Can you work these out from the model? Positions are in its coordinate system, mm. A direction names the side the tool comes from. Coordinates: 2 decimals unless noted, no trailing zeros. Order: outer loops, then holes, each group sorted by start corner. A loop starts at its lowest first (then second) coordinate and runs counter-clockwise, first axis right, second up. Notation, with made-up numbers: (5.25, -30.5) -> (19.25, -30.5) arc R27 cw to (19.25, -1.5) -> close; hole circle Ø3 at (36.25, 83). An arc over 180 degrees is marked (long way). Answer as a JSON object with one key per item and string values. Group by question number.
(1) I want a section at B-B, the plane x = -106. List the corners of the cut face in (y, z) for me, plus the area to 3 significant figures.
(2) If we mould it in two halves opening along X, with no side actions, what happens to faces 4 (the cylindrical face through (-622.038, 0.279, 0.178)), 5 (the flat face through (0, -5.4, 3.64)), 6 (the flat face through (-640, 17, 12.7))? For each: pulls with the +X half, pulls with the -X half, needs draft (parallel to the pull), parting line crosses it, or undercut.
(3) I need wall thicknesses on line 1 (X direction, y = -15, z = 7); line 2 (X direction, y = 7, z = -3.5); line 3 (X direction, y = 7, z = -1.5) (3 decimals). Which ranges of each line are inside material? Lowest first, please.
(4) For pin 1 (4 mm diameter, centred on x = 5, z = -3.5, fed in from -Y); pin 2 (4 mm diameter, centred on y = -14.5, z = -9, fed in from +X); pin 3 (2 mm diameter, centred on x = -356, z = 4, fed in from -Y), each with a flat end and sliding along its axis, tell me the tip position at first contact or that it passes through.
(5) Which directions (+Z, -Z, +X, -X, +Y, -Y) give clear straight access to the entire face, cutting with the end or side of a thin tool? Please do faces 1 (the cylindrical face through (15.51, -11.07, 2.38)), 2 (the cylindrical face through (-300.53, -1.38, -6.2)), 3 (the flat face through (-658, -12.7, 0)).
from build123d import *

# Parameters (mm, degrees)
F0_R     = 6.35
F1_DEPTH = 609.6
F2_W     = 15.875
F2_H     = 15.875
F3_DEPTH = 15.875
F4_R     = 7.9375
F5_DEPTH = 6.35
F6_R     = 6.35
F8_DEPTH = 12.7
F9_R     = 9.525
F10_R    = 3.175


with BuildPart() as f1:
    # F0 (on Right) → F1 (new body)
    with BuildSketch(Plane.YZ):
        Circle(F0_R)
    extrude(amount=-F1_DEPTH)

    # F2 (on Right) → F3 (join)
    with BuildSketch(Plane.YZ):
        Rectangle(F2_W, F2_H)
    extrude(amount=F3_DEPTH)

    # F4 (on face) → F5 (join)
    with BuildSketch(Plane.XZ.offset(7.9375)):
        with Locations((7.9375, 0)):
            Circle(F4_R)
    extrude(amount=F5_DEPTH)

    # F6
    f6_edges = [f1.edges().sort_by_distance(p)[0] for p in [
        (15.875, 0, 7.9375),
        (15.875, 0, -7.9375),
    ]]
    fillet(f6_edges, radius=F6_R)

    # F7 (on Top) → F8 (join, symmetric)
    with BuildSketch(Plane.XY):
        with BuildLine():
            Line((-609.6, -25.4), (-609.6, 25.4))
            Line((-609.6, 25.4), (-685.8, 25.4))
            Line((-685.8, 25.4), (-685.8, 12.7))
            Line((-685.8, 12.7), (-634.7345113754, 12.7))
            ThreePointArc((-634.7345113754, 12.7), (-622.0345113754, 0), (-634.7345113754, -12.7))
            Line((-634.7345113754, -12.7), (-685.8, -12.7))
            Line((-685.8, -12.7), (-685.8, -25.4))
            Line((-685.8, -25.4), (-609.6, -25.4))
        make_face()
    extrude(amount=F8_DEPTH, both=True)

    # F9
    f9_edges = [f1.edges().sort_by_distance(p)[0] for p in [
        (-609.6, 25.4, 0),
        (-609.6, -25.4, 0),
    ]]
    fillet(f9_edges, radius=F9_R)

    # F10
    f10_edges = [f1.edges().sort_by_distance(p)[0] for p in [
        (-685.8, 25.4, 0),
        (-685.8, -25.4, 0),
        (-685.8, 12.7, 0),
        (-685.8, -12.7, 0),
    ]]
    fillet(f10_edges, radius=F10_R)


solid = f1.part
Computed values:
{
 "1": {"outline": "circle Ø12.7 at (0, 0)", "area": "127 mm2"},
 "2": {"face 4": "pulls with the -X half", "face 5": "undercut", "face 6": "needs draft"},
 "3": {"line 1": "x = -685.68 to -609.6", "line 2": "x = -624.14 to -609.6, 0 to 15.58", "line 3": "x = -624.138 to -609.6, 0 to 15.875"},
 "4": {"pin 1": "stops at y = -14.29", "pin 2": "stops at x = 11.66", "pin 3": "stops at y = -5.6"},
 "5": {"face 1": "-Y", "face 2": "none", "face 3": "+Z, -Z, -X"}
}
